Geometry check sheet. Reference: the model listing, model coordinates, mm. Face numbers are marked on the shaded views. A direction names the side the tool comes from. Coordinates: 2 decimals unless noted, no trailing zeros. Write each loop counter-clockwise with the first axis right and the second up, starting at its lowest first coordinate (ties: lowest second). Pieces come first, ordered by that corner, then holes. Notation, with made-up numbers: (49, -14) -> (61, -14) arc R10 cw to (61, 5) -> close; hole circle Ø1 at (15, 15.5). An arc over 180 degrees is marked (long way). Answer as CSV lines item,"result".
```python
from build123d import *

# Parameters (mm, degrees)
SKETCH1_R           = 33
EXTRUDE1_DEPTH      = 10
SKETCH2_R           = 27.25
EXTRUDE2_DEPTH      = 21
EXTRUDE3_DEPTH      = 12
SKETCH4_R           = 2.45
EXTRUDE4_DEPTH      = 36
SKETCH5_R           = 2.45
EXTRUDE5_DEPTH      = 38
EXTRUDE5_DEPTH_BACK = 38
SKETCH6_W           = 19.894607887
SKETCH6_H           = 28
EXTRUDE6_DEPTH      = 12
SKETCH8_R           = 5.25
EXTRUDE7_DEPTH      = 26


with BuildPart() as part:
    # Sketch1 → Extrude1 (new body)
    with BuildSketch(Plane.XY):
        Circle(SKETCH1_R)
    extrude(amount=EXTRUDE1_DEPTH)

    # Sketch2 → Extrude2 (add)
    with BuildSketch(Plane.XY.offset(10)):
        Circle(SKETCH2_R)
    extrude(amount=EXTRUDE2_DEPTH)

    # Sketch3 → Extrude3 (cut)
    with BuildSketch(Plane.XY.offset(31)):
        with BuildLine():
            Line((-10.25, 11.291589791), (-10.25, -11.291589791))
            ThreePointArc((-10.25, -11.291589791), (0, -15.25), (10.25, -11.291589791))
            Line((10.25, -11.291589791), (10.25, 11.291589791))
            ThreePointArc((10.25, 11.291589791), (0, 15.25), (-10.25, 11.291589791))
        make_face()
    extrude(amount=-EXTRUDE3_DEPTH, mode=Mode.SUBTRACT)

    # Sketch4 → Extrude4 (cut)
    with BuildSketch(Plane(origin=(0, 0, 0), x_dir=(-1, 0, 0), z_dir=(0, 0, -1))):
        with Locations((0, 27.5)):
            Circle(SKETCH4_R)
        with Locations((-27.5, 0)):
            Circle(SKETCH4_R)
        with Locations((0, -27.5)):
            Circle(SKETCH4_R)
        with Locations((27.5, 0)):
            Circle(SKETCH4_R)
    extrude(amount=-EXTRUDE4_DEPTH, mode=Mode.SUBTRACT)

    # Sketch5 → Extrude5 (cut, two sides)
    with BuildSketch(Plane.ZY.offset(-10.25)) as extrude5_sk:
        with Locations((25.5, 6.5)):
            Circle(SKETCH5_R)
        with Locations((25.5, -6.5)):
            Circle(SKETCH5_R)
    extrude(amount=EXTRUDE5_DEPTH, mode=Mode.SUBTRACT)
    extrude(extrude5_sk.sketch, amount=-EXTRUDE5_DEPTH_BACK, mode=Mode.SUBTRACT)

    # Sketch6 → Extrude6 (cut)
    with BuildSketch(Plane.XY.offset(31)):
        with Locations((-26.197303943, 0)):
            Rectangle(SKETCH6_W, SKETCH6_H)
    extrude6 = extrude(amount=-EXTRUDE6_DEPTH, mode=Mode.SUBTRACT)

    # Mirror1: Extrude6 across plane
    add(extrude6.mirror(Plane(origin=(0, 0, 0), x_dir=(0, 0, 1), z_dir=(1, 0, 0))), mode=Mode.SUBTRACT)

    # Sketch8 → Extrude7 (cut)
    with BuildSketch(Plane.XY.offset(31)):
        with Locations((0, 27.5)):
            Circle(SKETCH8_R)
        with Locations((27.5, 0)):
            Circle(SKETCH8_R)
        with Locations((-27.5, 0)):
            Circle(SKETCH8_R)
        with Locations((0, -27.5)):
            Circle(SKETCH8_R)
    extrude(amount=-EXTRUDE7_DEPTH, mode=Mode.SUBTRACT)


solid = part.part
```
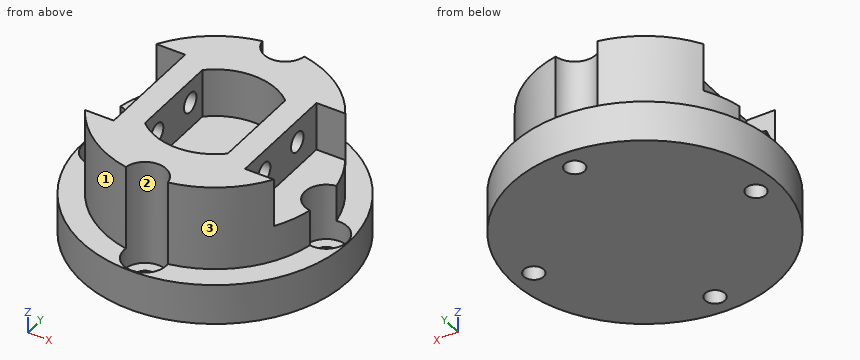
Item 1: Set-up check for the marked faces 1, 2 and 3: record each of +Z, -Z, +X, -X, +Y, -Y from which the full face is reachable in a straight line by a thin tool's end or side.
Responses:
face 1,"+Z, -X, -Y"
face 2,"+Z"
face 3,"+Z, +X, -Y"
Item 2: Thickness scan on probe 1 along Z at (x, y) = (-14.5, -6.5); probe 2 along Y at (x, z) = (-14.6, 25.5); probe 3 along Z at (x, y) = (-26, -12). Record the ranges inside material, lowest first.
Responses:
probe 1,"z = 0 to 23.05, 27.95 to 31"
probe 2,"y = -23.01 to -8.95, -4.05 to 4.05, 8.95 to 23.01"
probe 3,"z = 0 to 10"
Item 3: Cross-section at C-C, the plane z = 11. Record the cut outline in (x, y).
Responses:
outline,"(-26.75, -5.2) arc R27.25 ccw to (-5.2, -26.75) arc R5.25 cw to (5.2, -26.75) arc R27.25 ccw to (26.75, -5.2) arc R5.25 cw to (26.75, 5.2) arc R27.25 ccw to (5.2, 26.75) arc R5.25 cw to (-5.2, 26.75) arc R27.25 ccw to (-26.75, 5.2) arc R5.25 cw to start"
Item 4: Cross-section at A-A, the plane x = 0. Record the cut outline in (y, z), plus the area to 3 significant figures.
Responses:
outline,"(-33, 0) -> (-29.95, 0) -> (-29.95, 5) -> (-32.75, 5) -> (-32.75, 10) -> (-33, 10) -> close; (-25.05, 0) -> (25.05, 0) -> (25.05, 5) -> (22.25, 5) -> (22.25, 31) -> (15.25, 31) -> (15.25, 19) -> (-15.25, 19) -> (-15.25, 31) -> (-22.25, 31) -> (-22.25, 5) -> (-25.05, 5) -> close; (29.95, 0) -> (33, 0) -> (33, 10) -> (32.75, 10) -> (32.75, 5) -> (29.95, 5) -> close"
area,"1,070 mm2"
Item 5: Cross-section at D-D, the plane z = 4. Record the cut outline in (x, y).
Responses:
outline,"circle Ø66 at (0, 0); hole circle Ø4.9 at (-27.5, 0); hole circle Ø4.9 at (0, -27.5); hole circle Ø4.9 at (0, 27.5); hole circle Ø4.9 at (27.5, 0)"
Item 6: Depth check by flat-ended pin: pin 1 Ø5 at (x, y) = (27, 2) entering from +Z; pin 2 Ø2 at (x, z) = (20.5, 23) entering from -Y; pin 3 Ø2 at (x, z) = (-20.5, 25.5) entering from +Y. Enter the tip coordinate at first touch or a pass-through.
Responses:
pin 1,"stops at z = 5"
pin 2,"stops at y = -19.03"
pin 3,"stops at y = 19.03"
Item 7: Cross-section at B-B, the plane y = 0. Record the cut outline in (x, z), plus the area to 3 significant figures.
Responses:
outline,"(-33, 0) -> (-29.95, 0) -> (-29.95, 5) -> (-32.75, 5) -> (-32.75, 10) -> (-33, 10) -> close; (-25.05, 0) -> (25.05, 0) -> (25.05, 5) -> (22.25, 5) -> (22.25, 19) -> (16.25, 19) -> (16.25, 31) -> (10.25, 31) -> (10.25, 19) -> (-10.25, 19) -> (-10.25, 31) -> (-16.25, 31) -> (-16.25, 19) -> (-22.25, 19) -> (-22.25, 5) -> (-25.05, 5) -> close; (29.95, 0) -> (33, 0) -> (33, 10) -> (32.75, 10) -> (32.75, 5) -> (29.95, 5) -> close"
area,"1,050 mm2"
